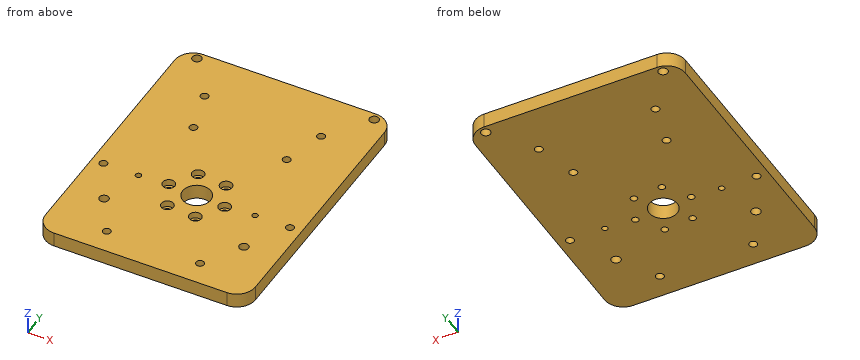
from build123d import *

# Parameters (mm, degrees)
DISCO_1_4IN_START                         = 83.85
DISCO_1_4IN_DEPTH                         = 6.35
BARRENOS_M1_ARO_ESCUADRAS_PASADORES_START = 83.85
CROQUIS16_R                               = 1.45
CROQUIS16_R_2                             = 1.25
CROQUIS16_R_3                             = 6
CROQUIS16_R_4                             = 2
BARRENOS_M1_ARO_ESCUADRAS_PASADORES_DEPTH = 6.35
REFRENTADO_M2_5_START                     = 87.4
CROQUIS17_R                               = 2.6
REFRENTADO_M2_5_DEPTH                     = 2.8
PASO_M3_ESCUADRAS_TUERCA_START            = 83.85
CROQUIS18_R                               = 1.7
PASO_M3_ESCUADRAS_TUERCA_DEPTH            = 6.35
PASO_M3_ARO_TUERCA_START                  = 83.85
CROQUIS19_R                               = 1.7
PASO_M3_ARO_TUERCA_DEPTH                  = 6.35


with BuildPart() as part:
    # Croquis15 → Disco_1-4in (new body)
    with BuildSketch(Plane.XY.offset(DISCO_1_4IN_START)):
        with BuildLine():
            Line((-37, -45), (37, -45))
            ThreePointArc((37, -45), (42.656854249, -42.656854249), (45, -37))
            Line((45, -37), (45, 66.2))
            ThreePointArc((45, 66.2), (42.656854249, 71.856854249), (37, 74.2))
            Line((37, 74.2), (-37, 74.2))
            ThreePointArc((-37, 74.2), (-42.656854249, 71.856854249), (-45, 66.2))
            Line((-45, 66.2), (-45, -37))
            ThreePointArc((-45, -37), (-42.656854249, -42.656854249), (-37, -45))
        make_face()
    extrude(amount=DISCO_1_4IN_DEPTH)

    # Croquis16 → Barrenos_M1_aro_escuadras_pasadores (cut)
    with BuildSketch(Plane.XY.offset(BARRENOS_M1_ARO_ESCUADRAS_PASADORES_START)):
        with Locations(Location((7.026042223, 10.338507178, 0), (0, 0, 180))):
            Circle(CROQUIS16_R)
        with Locations(Location((-5.440388742, 11.253984643, 0), (0, 0, 180))):
            Circle(CROQUIS16_R)
        with Locations(Location((-12.466430965, 0.915477464, 0), (0, 0, 180))):
            Circle(CROQUIS16_R)
        with Locations(Location((-7.026042223, -10.338507178, 0), (0, 0, 180))):
            Circle(CROQUIS16_R)
        with Locations(Location((5.440388742, -11.253984643, 0), (0, 0, 180))):
            Circle(CROQUIS16_R)
        with Locations(Location((12.466430965, -0.915477464, 0), (0, 0, 180))):
            Circle(CROQUIS16_R)
        with Locations(Location((40, 0, 0), (0, 0, 180))):
            Circle(CROQUIS16_R_2)
        with Locations(Location((20, 34.641016151, 0), (0, 0, 180))):
            Circle(CROQUIS16_R_2)
        with Locations(Location((-20, 34.641016151, 0), (0, 0, 180))):
            Circle(CROQUIS16_R_2)
        with Locations(Location((-40, 0, 0), (0, 0, 180))):
            Circle(CROQUIS16_R_2)
        with Locations(Location((-20, -34.641016151, 0), (0, 0, 180))):
            Circle(CROQUIS16_R_2)
        with Locations(Location((20, -34.641016151, 0), (0, 0, 180))):
            Circle(CROQUIS16_R_2)
        with Locations(Location((0, 0, 0), (0, 0, 180))):
            Circle(CROQUIS16_R_3)
        with Locations(Location((-25, 52.85, 0), (0, 0, 180))):
            Circle(CROQUIS16_R_2)
        with Locations(Location((-25, 0, 0), (0, 0, 180))):
            Circle(CROQUIS16_R_2)
        with Locations(Location((25, 52.85, 0), (0, 0, 180))):
            Circle(CROQUIS16_R_2)
        with Locations(Location((25, 0, 0), (0, 0, 180))):
            Circle(CROQUIS16_R_2)
        with Locations(Location((-38, 71.025, 0), (0, 0, 180))):
            Circle(CROQUIS16_R_4)
        with Locations(Location((38, 71.025, 0), (0, 0, 180))):
            Circle(CROQUIS16_R_4)
        with Locations(Location((-30, -18.175, 0), (0, 0, 180))):
            Circle(CROQUIS16_R_4)
        with Locations(Location((30, -18.175, 0), (0, 0, 180))):
            Circle(CROQUIS16_R_4)
    extrude(amount=BARRENOS_M1_ARO_ESCUADRAS_PASADORES_DEPTH, mode=Mode.SUBTRACT)

    # Croquis17 → Refrentado_M2-5 (cut)
    with BuildSketch(Plane.XY.offset(REFRENTADO_M2_5_START)):
        with Locations(Location((7.026042223, 10.338507178, 0), (0, 0, 180))):
            Circle(CROQUIS17_R)
        with Locations(Location((-5.440388742, 11.253984643, 0), (0, 0, 180))):
            Circle(CROQUIS17_R)
        with Locations(Location((-12.466430965, 0.915477464, 0), (0, 0, 180))):
            Circle(CROQUIS17_R)
        with Locations(Location((-7.026042223, -10.338507178, 0), (0, 0, 180))):
            Circle(CROQUIS17_R)
        with Locations(Location((5.440388742, -11.253984643, 0), (0, 0, 180))):
            Circle(CROQUIS17_R)
        with Locations(Location((12.466430965, -0.915477464, 0), (0, 0, 180))):
            Circle(CROQUIS17_R)
    extrude(amount=REFRENTADO_M2_5_DEPTH, mode=Mode.SUBTRACT)

    # Croquis18 → Paso_M3_escuadras_tuerca (cut)
    with BuildSketch(Plane.XY.offset(PASO_M3_ESCUADRAS_TUERCA_START)):
        with Locations(Location((-25, 52.85, 0), (0, 0, 180))):
            Circle(CROQUIS18_R)
        with Locations(Location((25, 52.85, 0), (0, 0, 180))):
            Circle(CROQUIS18_R)
    extrude(amount=PASO_M3_ESCUADRAS_TUERCA_DEPTH, mode=Mode.SUBTRACT)

    # Croquis19 → Paso_M3_aro_tuerca (cut)
    with BuildSketch(Plane.XY.offset(PASO_M3_ARO_TUERCA_START)):
        with Locations(Location((40, 0, 0), (0, 0, 180))):
            Circle(CROQUIS19_R)
        with Locations(Location((20, 34.641016151, 0), (0, 0, 180))):
            Circle(CROQUIS19_R)
        with Locations(Location((-20, 34.641016151, 0), (0, 0, 180))):
            Circle(CROQUIS19_R)
        with Locations(Location((-40, 0, 0), (0, 0, 180))):
            Circle(CROQUIS19_R)
        with Locations(Location((-20, -34.641016151, 0), (0, 0, 180))):
            Circle(CROQUIS19_R)
        with Locations(Location((20, -34.641016151, 0), (0, 0, 180))):
            Circle(CROQUIS19_R)
    extrude(amount=PASO_M3_ARO_TUERCA_DEPTH, mode=Mode.SUBTRACT)


solid = part.part
Could you check a few things on this model? Use its own coordinates, in mm. Coordinates: 2 decimals unless noted, no trailing zeros. Write each loop counter-clockwise with the first axis right and the second up, starting at its lowest first coordinate (ties: lowest second). Pieces come first, ordered by that corner, then holes. Notation, with made-up numbers: (20, -3) - (59, -3) arc R22 ccw to (59, 14) - close; hole circle Ø5 at (82, 14). An arc over 180 degrees is marked (long way). Write item = value, one per line.
1) Suppose I cut it at B-B on x = 25. Please give me the cut outline in (y, z), plus the area to 3 significant figures.
Result set:
outline = (-45, 83.85) - (-1.25, 83.85) - (-1.25, 90.2) - (-45, 90.2) - close; (1.25, 83.85) - (51.15, 83.85) - (51.15, 90.2) - (1.25, 90.2) - close; (54.55, 83.85) - (74.2, 83.85) - (74.2, 90.2) - (54.55, 90.2) - close
area = 719 mm2
2) Will these pins go through, and if not, where does the flat tip stop? pin 1 Ø2 at (x, y) = (-25, 0) entering from -Z; pin 2 Ø1.6 at (x, y) = (-6.5, 11.5) entering from +Z.
Result set:
pin_1 = through
pin_2 = 87.4
3) Suppose I cut it at C-C on z = 85.75. State how many separate pieces and enclosed holes the cut face has, plus the area to 3 significant figures.
Result set:
separate_pieces = 1
enclosed_holes = 21
area = 10,400 mm2
4) Suppose I cut it at A-A on x = -30. Please give me the cut outline in (y, z) (3 decimals).
Result set:
outline = (-45, 83.85) - (-20.175, 83.85) - (-20.175, 90.2) - (-45, 90.2) - close; (-16.175, 83.85) - (74.2, 83.85) - (74.2, 90.2) - (-16.175, 90.2) - close
5) Please list where these lines run through material, in increasing order: line 1 (Y direction, x = 25, z = 88.5); line 2 (Y direction, x = -20, z = 85); line 3 (X direction, y = 10, z = 89.5). Write a range as [from, to].
Result set:
line_1 = [-45, -1.25], [1.25, 51.15], [54.55, 74.2]
line_2 = [-45, -36.34], [-32.94, 32.94], [36.34, 74.2]
line_3 = [-45, -7.72], [-3.16, 4.45], [9.6, 45]
6) Suppose I cut it at D-D on x = -1.5. Please give me the cut outline in (y, z).
Result set:
outline = (-45, 83.85) - (-5.81, 83.85) - (-5.81, 90.2) - (-45, 90.2) - close; (5.81, 83.85) - (74.2, 83.85) - (74.2, 90.2) - (5.81, 90.2) - close
